from build123d import *

# Parameters (mm, degrees)
F0_W          = 10
F0_H          = 9
F0_R          = 1.85
F1_DEPTH      = 5
F5_ANGLE_BACK = 20
F5_ANGLE      = 40
F6_W          = 7
F6_H          = 1.5
F7_DEPTH      = 4
F8_W          = 0.2
F8_H          = 4
F9_DEPTH      = 25
F10_COUNT     = 2


with BuildPart() as f1:
    # F0 (on Top) → F1 (new body)
    with BuildSketch(Plane.XY):
        with Locations((5, -4.5)):
            Rectangle(F0_W, F0_H)
        with Locations((5, -4.5)):
            Circle(F0_R, mode=Mode.SUBTRACT)
    extrude(amount=F1_DEPTH)

    # F6 (on face) → F7 (join)
    with BuildSketch(Plane.XY.offset(5)):
        with Locations((4.5, -8.25)):
            Rectangle(F6_W, F6_H)
        with Locations((4.5, -0.75)):
            Rectangle(F6_W, F6_H)
    extrude(amount=F7_DEPTH)

    # F8 (on face) → F9 (cut)
    with BuildSketch(Plane.YZ.offset(10)):
        with Locations((-7.6, 7)):
            Rectangle(F8_W, F8_H)
        with Locations((-8.9, 7)):
            Rectangle(F8_W, F8_H)
        with Locations((-0.1, 7)):
            Rectangle(F8_W, F8_H)
        with Locations((-1.4, 7)):
            Rectangle(F8_W, F8_H)
    extrude(amount=-F9_DEPTH, mode=Mode.SUBTRACT)



with BuildPart() as f5:
    # F3 (on offset) → F5 (revolve)
    with BuildSketch(Plane.XZ.offset(4.5), mode=Mode.PRIVATE) as f5_sk:
        with BuildLine():
            Line((0.5, 5), (0, 5))
            Line((0, 5), (-0.5, 5))
            Line((-0.5, 5), (-0.5, 0))
            add(Edge.make_bspline(
                [(-0.5, 0), (-0.7940392474, -1.8718490053), (-2.3993364256, -10.2948176613), (-9.1089938236, -15.538515672), (-10.3149545762, -17)],
                knots=[0, 0, 0, 0, 0.5, 1, 1, 1, 1], degree=3))
            ThreePointArc((-10.3149545762, -17), (-10.1685444147, -17.5464101615), (-9.6221342532, -17.4))
            add(Edge.make_bspline(
                [(-9.6221342532, -17.4), (-8.3348966668, -15.9883498775), (-1.3566520207, -10.8349816991), (0.0036717937, -2.0199950425), (0.5, 0)],
                knots=[0, 0, 0, 0, 0.4942337757, 1, 1, 1, 1], degree=3))
            Line((0.5, 0), (0.5, 5))
        make_face()
    revolve(f5_sk.sketch.rotate(Axis((-20, -4.5, 1.4354154991), (0, 0, -1)), -F5_ANGLE_BACK), axis=Axis((-20, -4.5, 1.4354154991), (0, 0, -1)), revolution_arc=F5_ANGLE)


with BuildPart() as f1_1:
    add(f1.part)

    add(f5.part)  # F10 merges F5
    # F10: F5 ×2 about axis
    f10_axis = Axis((5, -4.5, 0), (0, 0, -1))
    for i in range(1, F10_COUNT):
        add(f5.part.rotate(f10_axis, i * 360 / F10_COUNT))


solid = f1_1.part
The listing builds one solid part. Answer for the finished solid, in the listing's coordinates (mm). A direction names the side the tool comes from. Give positions to 0.01 mm unless a question says otherwise; leave off trailing zeros. Write each loop counter-clockwise with the first axis right and the second up, starting at its lowest first coordinate (ties: lowest second). Pieces come first, ordered by that corner, then holes. Notation, with made-up numbers: (6, -4.75) - (11, -4.75) arc R17 ccw to (11, 28.25) - close; hole circle Ø10 at (42.5, -16.75). An arc over 180 degrees is marked (long way). Use a Markdown table: item, result.
1. For a pull along Y with two mould halves and no side action, classify faces 1 (the flat face through (4, -8, 9)), 2 (the flat face through (5, -7.7, 7)), 3 (the flat face through (-3.6, 1.47, -7.92)), 4 (the cylindrical face through (-0.5, -4.4, 2.5)) as released by +Y, released by -Y, zero draft, split by the parting line, or undercut.
Values follow:
| item | result |
|---|---|
| face 1 | zero draft |
| face 2 | undercut |
| face 3 | released by +Y |
| face 4 | undercut |
2. Find the intervals of material crossed by probe 1 along Y at (x, z) = (5, 3.55); probe 2 along Y at (x, z) = (1.5, 6); probe 3 along Z at (x, y) = (8, -4), in increasing order. Write a range as from..to.
Values follow:
| item | result |
|---|---|
| probe 1 | y = -9..-6.35, -2.65..0 |
| probe 2 | y = -8.8..-7.7, -1.3..-0.2 |
| probe 3 | z = 0..5 |
3. Section A-A on x = 5 is taken. Write down the section's boundary in (y, z), plus the area to 3 significant figures.
Values follow:
| item | result |
|---|---|
| outline | (-9, 0) - (-6.35, 0) - (-6.35, 5) - (-7.7, 5) - (-7.7, 9) - (-8.8, 9) - (-8.8, 5) - (-9, 5) - close; (-2.65, 0) - (0, 0) - (0, 5) - (-0.2, 5) - (-0.2, 9) - (-1.3, 9) - (-1.3, 5) - (-2.65, 5) - close |
| area | 35.3 mm² |
4. A tool of negligible diameter and unlimited length cuts with its end or side. For faces 5 (the flat face through (8, -8, 7)), 6 (the flat face through (5, -8.8, 7)), 7 (the cylindrical face through (10.5, -4.6, 2.5)), from which of +Z, -Z, +X, -X, +Y, -Y can it reach the whole face along a straight path? Write none if from no direction.
Values follow:
| item | result |
|---|---|
| face 5 | +Z, +X, +Y, -Y |
| face 6 | +Z, +X, -X, -Y |
| face 7 | +Z, +X |
5. Each of these flat-tipped pins is pushed along its axis until it touches: P1, Ø4, axis at y = -9.5, z = 4.5, coming from the +X side; P2, Ø1.5, axis at y = -7.5, z = -9.5, coming from the -X side; P3, Ø4.5, axis at x = 3.5, z = 8, coming from the -Y side; P4, Ø3.5, axis at x = 5, y = -4.5, coming from the -Z side. Where does it stop, or does it pass through?
Values follow:
| item | result |
|---|---|
| P1 | stops at x = 11.68 |
| P2 | stops at x = -4.47 |
| P3 | stops at y = -8.8 |
| P4 | passes through |
